Read the model definition and answer for the solid it produces. Units are mm, in the model's axes. A direction names the side the tool comes from. Give positions to 0.01 mm unless a question says otherwise; leave off trailing zeros. Write each loop counter-clockwise with the first axis right and the second up, starting at its lowest first coordinate (ties: lowest second). Pieces come first, ordered by that corner, then holes.
```python
from build123d import *

# Parameters (mm, degrees)
SALIENTE_EXTRUIR1_DEPTH = 147.5
CROQUIS2_R              = 0.25
SALIENTE_EXTRUIR2_DEPTH = 0.5


with BuildPart() as part:
    # Croquis1 → Saliente-Extruir1 (new body)
    with BuildSketch(Plane(origin=(0, 0, 0), x_dir=(0, 0, -1), z_dir=(1, 0, 0))):
        Polygon((0, 0), (134.5, 0), (134.5, 1), (-0.495643149, 1), (-16.116757416, -19.527932056), (-15.320966749, -20.133503865), align=None)
    extrude(amount=SALIENTE_EXTRUIR1_DEPTH)

    # Croquis2 → Saliente-Extruir2 (add)
    with BuildSketch(Plane(origin=(147.5, 0, 0), x_dir=(0, 0, -1), z_dir=(1, 0, 0))):
        with Locations(Location((134, 0.5, 0), (0, 0, 180))):
            Circle(CROQUIS2_R)
    extrude(amount=SALIENTE_EXTRUIR2_DEPTH)

    # Simetría1: part across plane


with BuildPart() as part_1:
    add(part.part)
    add(part.part.mirror(Plane.ZY))


solid = part_1.part
```
Item 1: Find the intervals of material crossed by line 1 along Y through (x, z) = (-12.5, -76); line 2 along Z through (x, y) = (24, -8.5); line 3 along Z through (x, y) = (31, -7.75), in increasing order.
Result set:
line 1: y = 0 to 1
line 2: z = 6.47 to 7.72
line 3: z = 5.9 to 7.15
Item 2: Section A-A (x = 92.5) is taken. Write down the section's boundary in (y, z).
Result set:
outline: (-20.13, 15.32) - (0, 0) - (0, -134.5) - (1, -134.5) - (1, 0.5) - (-19.53, 16.12) - close
Item 3: Which of the six approach directions +Z, -Z, +X, -X, +Y, -Y give full straight-line access (tool end or side, diameter ignored) to faces 1 (the flat face through (2, 0, -66)), 2 (the flat face through (2.065, -9.12, 8.197))?
Result set:
face 1: -Z, +X, -X, -Y
face 2: +Z, +X, -X, +Y
Item 4: Section B-B (z = -5.5) is taken. Write down the section's boundary in (x, y), and give its area (3 significant figures).
Result set:
outline: (-147.5, 0) - (147.5, 0) - (147.5, 1) - (-147.5, 1) - close
area: 295 mm2
Item 5: This flat-tipped pin is pushed along its axis until it touches: pin 1 Ø3 at (x, y) = (-101, -4) entering from -Z. Where does it stop, or does it pass through?
Result set:
pin 1: stops at z = 1.9
Item 6: Section C-C (y = -3.5) is taken. Write down the section's boundary in (x, z).
Result set:
outline: (-147.5, 2.66) - (147.5, 2.66) - (147.5, 3.92) - (-147.5, 3.92) - close
